For this review, take the finished solid that the model builds, in its own axes (mm). Round coordinates to 2 decimals unless told otherwise and drop trailing zeros. Write each loop counter-clockwise with the first axis right and the second up, starting at its lowest first coordinate (ties: lowest second). Pieces come first, ordered by that corner, then holes. Notation, with made-up numbers: M 86.5,52.25 L 90.5,52.25 A22 ccw 90.5,89.25 Z; hole C -35,74 d7. An arc over 180 degrees is marked long. Use one line per item in the form item = value. Start each with the question number.
Item 1: Add section A-A (z = -39.5). State the section outline as (x, y) points, and give its area (3 significant figures).
Item 2: For line 1 (Z direction, x = -0.5, y = 200); line 2 (Z direction, x = -1.25, y = 205); line 3 (Y direction, x = -1, z = -388), list the stretches that pass through material, from the lowest coordinate up. Write a range as [from, to].
Item 3: For P1, Ø1.5, axis at x = -2.5, y = 76.5, coming from the +Z side, flat-tipped, find the tip position at first contact; note if it passes through.
Item 4: Add section B-B (y = 187.5). State the section outline as (x, z) points.
from build123d import *

# Parameters (mm, degrees)
BASE_FLANGE1_DEPTH = 2.588


# Sheet-metal steps are written as plain solids
with BuildPart() as part:
    # Base-Flange1: sheet metal written as solids
    # Sketch1 → Base-Flange1 (new body)
    with BuildSketch(Plane(origin=(0, 0, 0), x_dir=(0, 0, -1), z_dir=(1, 0, 0))):
        Polygon((0, 172), (85.688880405, 232), (371.300951546, 232), (475.224, 172), (475.224, 0), (0, 0), align=None)
    extrude(amount=-BASE_FLANGE1_DEPTH)

    # Fillet1
    # a fillet whose section is not a circle: 25 mm, written as the material it takes off along each edge
    with BuildSketch(Plane(origin=(19.706174305, 232, -85.688880405), x_dir=(0, -0.5735764363510439, 0.8191520442889934), z_dir=(-1, 0, 0))) as fillet1_piece_1:
        with BuildLine():
            add(Edge.make_bspline([(7.882469722, 0), (6.425514187, 0), (4.968558652, 0), (1.72149306, -0.207126843), (-1.291361483, -1.157076231), (-4.070004977, -2.849848165), (-5.263473082, -3.685523529), (-6.456941187, -4.521198893)], knots=[0, 0, 0, 0, 0, 0, 0.5, 0.5, 1, 1, 1, 1, 1, 1], degree=5))
            Line((-6.456941187, -4.521198893), (0, 0))
            Line((0, 0), (7.882469722, 0))
        make_face()
    extrude(amount=42.00034861, mode=Mode.SUBTRACT)
    with BuildSketch(Plane(origin=(16.746824527, 232, -371.300951546), x_dir=(0, 0, 1), z_dir=(-1, 0, 0))) as fillet1_piece_2:
        with BuildLine():
            add(Edge.make_bspline([(6.698729811, 0), (5.455779776, 0), (4.212829741, 0), (1.444392876, -0.149716053), (-1.176022897, -0.851854343), (-3.648417578, -2.106414871), (-4.724843884, -2.727889888), (-5.801270189, -3.349364905)], knots=[0, 0, 0, 0, 0, 0, 0.5, 0.5, 1, 1, 1, 1, 1, 1], degree=5))
            Line((-5.801270189, -3.349364905), (0, 0))
            Line((0, 0), (6.698729811, 0))
        make_face()
    extrude(amount=36.081649054, mode=Mode.SUBTRACT)


solid = part.part
Calculated:
q1.outline = M -2.59,0 L 0,0 L 0,199.66 L -2.59,199.66 Z
q1.area = 517 mm^2
q2.line_1 = [-426.73, -39.99]
q2.line_2 = [-418.07, -47.13]
q2.line_3 = [0, 222.36]
q3.P1 = 0
q4.outline = M -2.59,-448.38 L 0,-448.38 L 0,-22.14 L -2.59,-22.14 Z
